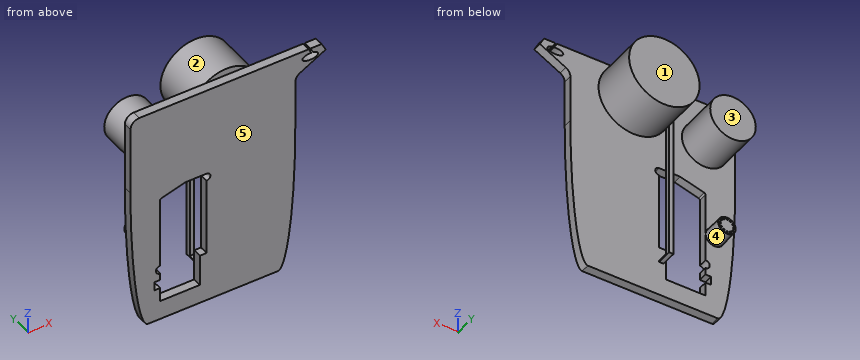
```python
from build123d import *

# Parameters (mm, degrees)
SKETCH1_W           = 9.4
SKETCH1_H           = 12.9
BOSS_EXTRUDE1_DEPTH = 0.5
FILLET4_R           = 0.5
FILLET7_R           = 0.5
FILLET8_SIZE        = 1
FILLET8_SIZE_2      = 8.5
FILLET9_SIZE        = 8.5
FILLET9_SIZE_2      = 1
SKETCH2_RX          = 0.452766649
SKETCH2_RY          = 0.2
CUT_EXTRUDE1_DEPTH  = 0.5
CUT_EXTRUDE2_DEPTH  = 0.5
CUT_EXTRUDE3_DEPTH  = 0.5
BOSS_EXTRUDE2_DEPTH = 0.25
SKETCH6_R           = 0.5
BOSS_EXTRUDE3_DEPTH = 0.7
SKETCH7_R           = 0.5
BOSS_EXTRUDE4_DEPTH = 0.4
DRAFT1_ANGLE        = 1
SKETCH17_R          = 0.05
CUT_EXTRUDE6_DEPTH  = 0.2
CIRPATTERN1_COUNT   = 12
CHAMFER3_SIZE       = 0.01
CHAMFER3_SIZE_2     = 0.010179202
SKETCH22_R          = 1.3
BOSS_EXTRUDE6_DEPTH = 2.5
SKETCH23_R          = 0.9
BOSS_EXTRUDE8_DEPTH = 0.7
SKETCH24_R          = 2.012011857
BOSS_EXTRUDE9_DEPTH = 2.7
FILLET12_R          = 0.1


with BuildPart() as part:
    # Sketch1 → Boss-Extrude1 (new body)
    with BuildSketch(Plane(origin=(0, 0, 0), x_dir=(1, 0, 0), z_dir=(0, 1, 0))):
        Polygon((0.065621543, 7.744296826), (0.065621543, 6.358511849), (1.565621543, 6.358511849), (1.804669866, 6.797665466), align=None)
        with Locations((-4.634378457, 12.808511849)):
            Rectangle(SKETCH1_W, SKETCH1_H)
    extrude(amount=BOSS_EXTRUDE1_DEPTH)

    # Fillet4
    fillet4_edges = [part.edges().sort_by_distance(p)[0] for p in [
        (0.065621543, 0.25, -7.744296826),
    ]]
    fillet(fillet4_edges, radius=FILLET4_R)

    # Fillet7
    fillet7_edges = [part.edges().sort_by_distance(p)[0] for p in [
        (-9.334378457, 0.25, -6.358511849),
    ]]
    fillet(fillet7_edges, radius=FILLET7_R)

    # Fillet8
    # an asymmetric fillet: 8.5, 1 mm, written as the material it takes off along each edge
    with BuildSketch(Plane(origin=(0.065621543, -21.25, -19.258511849), x_dir=(-1, 0, 0), z_dir=(0, 1, 0))) as fillet8_piece_1:
        with BuildLine():
            Bezier((FILLET8_SIZE, 0), (0, 0), (0, FILLET8_SIZE_2), weights=[1, 0.707106781, 1])
            Line((0, FILLET8_SIZE_2), (0, 0))
            Line((0, 0), (FILLET8_SIZE, 0))
        make_face()
    extrude(amount=43, mode=Mode.SUBTRACT)

    # Fillet9
    # an asymmetric fillet: 8.5, 1 mm, written as the material it takes off along each edge
    with BuildSketch(Plane(origin=(-9.334378457, -21.25, -19.258511849), x_dir=(0, 0, 1), z_dir=(0, 1, 0))) as fillet9_piece_1:
        with BuildLine():
            Bezier((FILLET9_SIZE, 0), (0, 0), (0, FILLET9_SIZE_2), weights=[1, 0.707106781, 1])
            Line((0, FILLET9_SIZE_2), (0, 0))
            Line((0, 0), (FILLET9_SIZE, 0))
        make_face()
    extrude(amount=43, mode=Mode.SUBTRACT)

    # Sketch2 → Cut-Extrude1 (cut)
    with BuildSketch(Plane(origin=(0, 0.5, 0), x_dir=(1, 0, 0), z_dir=(0, 1, 0))):
        with Locations(Location((0.922326291, 6.84128542), (0, 0, 180))):
            Ellipse(SKETCH2_RX, SKETCH2_RY)
    extrude(amount=-CUT_EXTRUDE1_DEPTH, mode=Mode.SUBTRACT)

    # Sketch3 → Cut-Extrude2 (cut)
    with BuildSketch(Plane(origin=(0, 0, 0), x_dir=(1, 0, 0), z_dir=(0, 1, 0))):
        Polygon((1.096292862, 6.656637946), (0.922326291, 6.358511849), (0.822326291, 6.358511849), (0.988590825, 6.643438984), align=None)
    extrude(amount=CUT_EXTRUDE2_DEPTH, mode=Mode.SUBTRACT)

    # Sketch4 → Cut-Extrude3 (cut)
    with BuildSketch(Plane(origin=(0, 0.5, 0), x_dir=(1, 0, 0), z_dir=(0, 1, 0))):
        with BuildLine():
            Line((-7.643596283, 18.158511849), (-7.643596283, 17.358511849))
            Line((-7.643596283, 17.358511849), (-7.970654201, 17.358511849))
            Line((-7.970654201, 17.358511849), (-7.970654201, 16.858511849))
            Line((-7.970654201, 16.858511849), (-7.643596283, 16.858511849))
            Line((-7.643596283, 16.858511849), (-7.643596283, 16.458511849))
            ThreePointArc((-7.643596283, 16.458511849), (-7.885861407, 16.216246725), (-7.643596283, 15.973981601))
            Line((-7.643596283, 15.973981601), (-7.643596283, 11.873981601))
            Line((-7.643596283, 11.873981601), (-6.193596283, 11.468418687))
            Line((-6.193596283, 11.468418687), (-4.993596283, 11.468418687))
            ThreePointArc((-4.993596283, 11.468418687), (-4.775557671, 11.686457299), (-4.993596283, 11.904495911))
            Line((-4.993596283, 11.904495911), (-4.993596283, 12.570725002))
            Line((-4.993596283, 12.570725002), (-4.993596283, 16.358511849))
            Line((-4.993596283, 16.358511849), (-5.378417371, 16.358511849))
            Line((-5.378417371, 16.358511849), (-5.378417371, 18.158511849))
            Line((-5.378417371, 18.158511849), (-7.643596283, 18.158511849))
        make_face()
    extrude(amount=-CUT_EXTRUDE3_DEPTH, mode=Mode.SUBTRACT)

    # Sketch5 → Boss-Extrude2 (add)
    with BuildSketch(Plane.ZY.offset(5)):
        with BuildLine():
            Line((-17.246848227, 0.5), (-17.246848227, 1.377441322))
            Line((-17.246848227, 1.377441322), (-8.88627879, 1.377441322))
            ThreePointArc((-8.88627879, 1.377441322), (-8.742131041, 1.233293573), (-8.88627879, 1.089145824))
            Line((-8.88627879, 1.089145824), (-17.164478085, 1.089145824))
            Line((-17.164478085, 1.089145824), (-17.164478085, 0.5))
            Line((-17.164478085, 0.5), (-17.246848227, 0.5))
        make_face()
    extrude(amount=BOSS_EXTRUDE2_DEPTH)

    # Sketch6 → Boss-Extrude3 (add)
    with BuildSketch(Plane(origin=(0, 0.5, 0), x_dir=(1, 0, 0), z_dir=(0, 1, 0))):
        with Locations(Location((-8.1644663, 14.36207626, 0), (0, 0, 270))):
            Circle(SKETCH6_R)
    extrude(amount=BOSS_EXTRUDE3_DEPTH)

    # Sketch7 → Boss-Extrude4 (add)
    with BuildSketch(Plane(origin=(0, 1.2, 0), x_dir=(1, 0, 0), z_dir=(0, 1, 0))):
        with Locations(Location((-8.1644663, 14.36207626, 0), (0, 0, 270))):
            Circle(SKETCH7_R)
    extrude(amount=BOSS_EXTRUDE4_DEPTH)

    # Draft1
    draft1_faces = [part.faces().sort_by_distance(p)[0] for p in [
        (-8.1644663, 1.05, -14.86207626),
    ]]
    draft(draft1_faces, Plane(origin=(-8.1644663, 1.6, -14.36207626), x_dir=(0, 0, 1), z_dir=(0, 1, 0)), DRAFT1_ANGLE)

    # Sketch17 → Cut-Extrude6 (cut)
    with BuildSketch(Plane(origin=(0, 1.6, 0), x_dir=(1, 0, 0), z_dir=(0, 1, 0))):
        with Locations(Location((-8.16651982, 14.750544579, 0), (0, 0, 270))):
            Circle(SKETCH17_R)
    cut_extrude6 = extrude(amount=-CUT_EXTRUDE6_DEPTH, mode=Mode.SUBTRACT)

    # CirPattern1: Cut-Extrude6 ×12 about axis
    cirpattern1_axis = Axis((-8.164445557, 0, -14.358152338), (0, 1, 0))
    for i in range(1, CIRPATTERN1_COUNT):
        add(cut_extrude6.rotate(cirpattern1_axis, i * 360 / CIRPATTERN1_COUNT), mode=Mode.SUBTRACT)

    # Chamfer3
    # the kernel refuses this chamfer: 0.010179202, 0.01 mm, written as the material it adds along each edge
    with BuildSketch(Plane(origin=(-8.1644663, 0.5, -14.36207626), x_dir=(0, 0, 1), z_dir=(-1, 0, 0))) as chamfer3_piece_1_section:
        Polygon((0.519200571 + CHAMFER3_SIZE, 0), (0.519200571 - CHAMFER3_SIZE_2 * 0.0174524062842, CHAMFER3_SIZE_2 * 0.999847686386), (0.519200571, 0), align=None)
    chamfer3_piece_1 = revolve(axis=Axis((-8.1644663, 0.5, -14.36207626), (0, 1, 0)), mode=Mode.PRIVATE)
    chamfer3_piece_1 = split(chamfer3_piece_1, bisect_by=Plane(origin=(-7.643596283, 0.504689418, -14.885788598), z_dir=(-1, 0, 0)), keep=Keep.TOP, mode=Mode.PRIVATE)
    add(chamfer3_piece_1)
    # the kernel refuses this chamfer: 0.010179202, 0.01 mm, written as the material it takes off along each edge
    with BuildSketch(Plane(origin=(-8.1644663, 1.6, -14.36207626), x_dir=(0, 0, 1), z_dir=(-1, 0, 0))) as chamfer3_2_piece_1:
        Polygon((0.5 + CHAMFER3_SIZE * 0.0174524064372, -CHAMFER3_SIZE * 0.999847695156), (0.5 - CHAMFER3_SIZE_2 * 0.999999991228, 0), (0.5, 0), align=None)
    revolve(axis=Axis((-8.1644663, 1.6, -14.36207626), (0, 1, 0)), mode=Mode.SUBTRACT)

    # Sketch22 → Boss-Extrude6 (add)
    with BuildSketch(Plane(origin=(0, 0.5, 0), x_dir=(1, 0, 0), z_dir=(0, 1, 0))):
        with Locations(Location((-7.597449318, 8.940947153, 0), (0, 0, 270))):
            Circle(SKETCH22_R)
    extrude(amount=BOSS_EXTRUDE6_DEPTH)

    # Sketch23 → Boss-Extrude8 (add)
    with BuildSketch(Plane(origin=(0, 0.5, 0), x_dir=(1, 0, 0), z_dir=(0, 1, 0))):
        with Locations(Location((-3.101125203, 8.659155236, 0), (0, 0, 270))):
            Circle(SKETCH23_R)
    extrude(amount=BOSS_EXTRUDE8_DEPTH)

    # Sketch24 → Boss-Extrude9 (add)
    with BuildSketch(Plane(origin=(0, 1.2, 0), x_dir=(1, 0, 0), z_dir=(0, 1, 0))):
        with Locations(Location((-3.101125203, 8.659155236, 0), (0, 0, 160.694494452))):
            Circle(SKETCH24_R)
    extrude(amount=BOSS_EXTRUDE9_DEPTH)

    # Fillet12
    fillet12_edges = [part.edges().sort_by_distance(p)[0] for p in [
        (-7.643596283, 0.25, -11.873981601),
    ]]
    fillet(fillet12_edges, radius=FILLET12_R)


solid = part.part
```
Read the model definition and answer for the solid it produces. Units are mm, in the model's axes. Face numbers are marked on the shaded views. A direction names the side the tool comes from. Give positions to 0.01 mm unless a question says otherwise; leave off trailing zeros. Order: outer loops, then holes, each group sorted by start corner. A loop starts at its lowest first (then second) coordinate and runs counter-clockwise, first axis right, second up.
(1) Given pin 1 (0.6 mm diameter, centred on y = 0, z = -13.5, fed in from -X); pin 2 (3 mm diameter, centred on x = 0, z = -14, fed in from +Y); pin 3 (2 mm diameter, centred on y = 3.5, z = -14.5, fed in from +X); pin 4 (0.8 mm diameter, centred on x = -8, z = -9.5, fed in from +Y), each flat-ended and moving along its own axis, determine where each tip first touches the part or whether it passes through.
(2) For the marked faces 1, 2 and 3, determine the directions among +Z, -Z, +X, -X, +Y, -Y from which every point of the face is accessible in a straight line to the end or side of a thin tool.
(3) Find section C-C (x = -3.25). Give the vertices of the cut face in (y, z).
(4) Straight lines are drawn through the part: L1, parallel to Y at x = -1.5, z = -7.5; L2, parallel to Y at x = -8, z = -15; L3, parallel to Z at x = -7.5, y = 1. For each, find the intervals that lie inside material, in ascending order.
(5) Find section B-B (y = 0.75). Give the vertices of the cut face in (x, z), plus the area to 3 significant figures.
(6) Find section D-D (y = 2.1). Give the vertices of the cut face in (x, z).
(7) Find section A-A (z = -9.75). Give the vertices of the cut face in (x, y).
(8) For a pull along Z with two mould halves and no side action, classify the marked faces 4 and 5 as released by +Z, released by -Z, zero draft, split by the parting line, or undercut.
Result sheet:
1. pin 1: stops at x = -9.29
1. pin 2: stops at y = 0.5
1. pin 3: passes through
1. pin 4: stops at y = 3
2. face 1: +Z, -Z, +X, -X, +Y
2. face 2: +Y
2. face 3: +Z, -Z, -X, +Y
3. outline: (0, -19.26) - (0.5, -19.26) - (0.5, -9.55) - (1.2, -9.55) - (1.2, -10.67) - (3.9, -10.67) - (3.9, -6.65) - (1.2, -6.65) - (1.2, -7.77) - (0.5, -7.77) - (0.5, -6.36) - (0, -6.36) - close
4. L1: y = 0 to 0.5, 1.2 to 3.9
4. L2: y = 0 to 0.5
4. L3: z = -10.24 to -7.64
5. outline: circle Ø2.6 at (-7.6, -8.94); circle Ø1.03 at (-8.16, -14.36); (-5.25, -17.25) - (-5, -17.25) - (-5, -17.16) - (-5.25, -17.16) - close; circle Ø1.8 at (-3.1, -8.66)
5. area: 8.71 mm2
6. outline: circle Ø2.6 at (-7.6, -8.94); circle Ø4.02 at (-3.1, -8.66)
7. outline: (-9.33, 0) - (0.07, 0) - (0.07, 0.5) - (-6.58, 0.5) - (-6.58, 3) - (-8.62, 3) - (-8.62, 0.5) - (-9.33, 0.5) - close; (-5.25, 1.09) - (-5, 1.09) - (-5, 1.38) - (-5.25, 1.38) - close; (-4.79, 1.2) - (-1.41, 1.2) - (-1.41, 3.9) - (-4.79, 3.9) - close
8. face 4: undercut
8. face 5: zero draft
